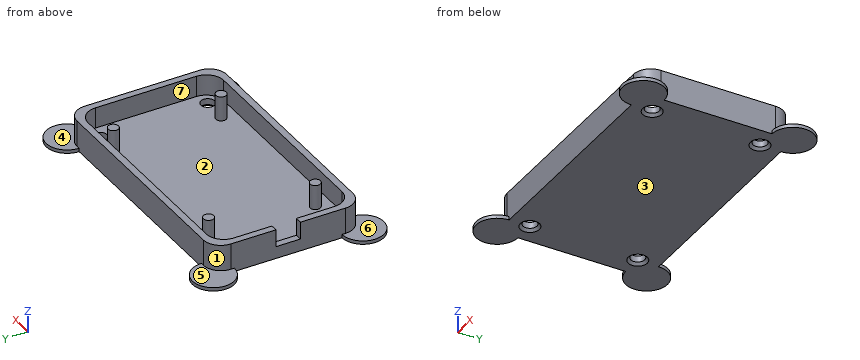
```python
from build123d import *

# Parameters (mm, degrees)
F0_R           = 2
F0_R_2         = 1.5
F0_W           = 2
F0_H           = 7
F1_DEPTH       = 2.5
F2_DEPTH       = 8.5
F3_DEPTH       = 9.6
F4_DEPTH       = 3.5
F5_D           = 3
F5_CSINK_D     = 5.5
F5_CSINK_ANGLE = 90
F6_DEPTH       = 1


with BuildPart() as f1:
    # F0 (on Top) → F1 (new body)
    with BuildSketch(Plane.XY):
        with BuildLine():
            Line((52.2425711751, 68.4110085815), (-6.7574288249, 68.4110085815))
            ThreePointArc((-6.7574288249, 68.4110085815), (-10.2929627308, 66.9465424875), (-11.7574288249, 63.4110085815))
            Line((-11.7574288249, 63.4110085815), (-11.7574288249, 52.4110085815))
            Line((-11.7574288249, 52.4110085815), (-11.7574288249, 45.4110085815))
            Line((-11.7574288249, 45.4110085815), (-11.7574288249, 34.4110085815))
            ThreePointArc((-11.7574288249, 34.4110085815), (-10.2929627308, 30.8754746756), (-6.7574288249, 29.4110085815))
            Line((-6.7574288249, 29.4110085815), (52.2425711751, 29.4110085815))
            ThreePointArc((52.2425711751, 29.4110085815), (55.778105081, 30.8754746756), (57.2425711751, 34.4110085815))
            Line((57.2425711751, 34.4110085815), (57.2425711751, 63.4110085815))
            ThreePointArc((57.2425711751, 63.4110085815), (55.778105081, 66.9465424875), (52.2425711751, 68.4110085815))
        make_face()
        with Locations((-7.7574288249, 33.4110085815)):
            Circle(F0_R, mode=Mode.SUBTRACT)
        with Locations((-1.2574288249, 33.9110085815)):
            Circle(F0_R_2, mode=Mode.SUBTRACT)
        with Locations((45.7425711751, 33.9110085815)):
            Circle(F0_R_2, mode=Mode.SUBTRACT)
        with Locations((53.2425711751, 33.4110085815)):
            Circle(F0_R, mode=Mode.SUBTRACT)
        with Locations((-7.7574288249, 64.4110085815)):
            Circle(F0_R, mode=Mode.SUBTRACT)
        with Locations((-1.8220887287, 64.9110085815)):
            Circle(F0_R_2, mode=Mode.SUBTRACT)
        with Locations((45.7425711751, 64.9110085815)):
            Circle(F0_R_2, mode=Mode.SUBTRACT)
        with Locations((53.2425711751, 64.4110085815)):
            Circle(F0_R, mode=Mode.SUBTRACT)
        with BuildLine():
            ThreePointArc((-11.7574288249, 63.4110085815), (-10.2929627308, 66.9465424875), (-6.7574288249, 68.4110085815))
            Line((-6.7574288249, 68.4110085815), (52.2425711751, 68.4110085815))
            ThreePointArc((52.2425711751, 68.4110085815), (55.778105081, 66.9465424875), (57.2425711751, 63.4110085815))
            Line((57.2425711751, 63.4110085815), (57.2425711751, 34.4110085815))
            ThreePointArc((57.2425711751, 34.4110085815), (55.778105081, 30.8754746756), (52.2425711751, 29.4110085815))
            Line((52.2425711751, 29.4110085815), (-6.7574288249, 29.4110085815))
            ThreePointArc((-6.7574288249, 29.4110085815), (-10.2929627308, 30.8754746756), (-11.7574288249, 34.4110085815))
            Line((-11.7574288249, 34.4110085815), (-11.7574288249, 45.4110085815))
            Line((-11.7574288249, 45.4110085815), (-13.7574288249, 45.4110085815))
            Line((-13.7574288249, 45.4110085815), (-13.7574288249, 33.4110085815))
            Line((-13.7574288249, 33.4110085815), (-13.7574288249, 32.4110085815))
            ThreePointArc((-13.7574288249, 32.4110085815), (-12.2929627308, 28.8754746756), (-8.7574288249, 27.4110085815))
            Line((-8.7574288249, 27.4110085815), (-7.7574288249, 27.4110085815))
            Line((-7.7574288249, 27.4110085815), (53.2425711751, 27.4110085815))
            Line((53.2425711751, 27.4110085815), (54.2425711751, 27.4110085815))
            ThreePointArc((54.2425711751, 27.4110085815), (57.778105081, 28.8754746756), (59.2425711751, 32.4110085815))
            Line((59.2425711751, 32.4110085815), (59.2425711751, 33.4110085815))
            Line((59.2425711751, 33.4110085815), (59.2425711751, 64.4110085815))
            Line((59.2425711751, 64.4110085815), (59.2425711751, 65.4110085815))
            ThreePointArc((59.2425711751, 65.4110085815), (57.778105081, 68.9465424875), (54.2425711751, 70.4110085815))
            Line((54.2425711751, 70.4110085815), (53.2425711751, 70.4110085815))
            Line((53.2425711751, 70.4110085815), (-7.7574288249, 70.4110085815))
            Line((-7.7574288249, 70.4110085815), (-8.7574288249, 70.4110085815))
            ThreePointArc((-8.7574288249, 70.4110085815), (-12.2929627308, 68.9465424875), (-13.7574288249, 65.4110085815))
            Line((-13.7574288249, 65.4110085815), (-13.7574288249, 64.4110085815))
            Line((-13.7574288249, 64.4110085815), (-13.7574288249, 52.4110085815))
            Line((-13.7574288249, 52.4110085815), (-11.7574288249, 52.4110085815))
            Line((-11.7574288249, 52.4110085815), (-11.7574288249, 63.4110085815))
        make_face()
        with Locations((-1.2574288249, 33.9110085815)):
            Circle(F0_R_2)
        with Locations((45.7425711751, 33.9110085815)):
            Circle(F0_R_2)
        with Locations((45.7425711751, 64.9110085815)):
            Circle(F0_R_2)
        with Locations((-1.8220887287, 64.9110085815)):
            Circle(F0_R_2)
        with Locations((-12.7574288249, 48.9110085815)):
            Rectangle(F0_W, F0_H)
    extrude(amount=F1_DEPTH)

    # F0 (on Top) → F2 (join)
    with BuildSketch(Plane.XY):
        with BuildLine():
            ThreePointArc((-11.7574288249, 63.4110085815), (-10.2929627308, 66.9465424875), (-6.7574288249, 68.4110085815))
            Line((-6.7574288249, 68.4110085815), (52.2425711751, 68.4110085815))
            ThreePointArc((52.2425711751, 68.4110085815), (55.778105081, 66.9465424875), (57.2425711751, 63.4110085815))
            Line((57.2425711751, 63.4110085815), (57.2425711751, 34.4110085815))
            ThreePointArc((57.2425711751, 34.4110085815), (55.778105081, 30.8754746756), (52.2425711751, 29.4110085815))
            Line((52.2425711751, 29.4110085815), (-6.7574288249, 29.4110085815))
            ThreePointArc((-6.7574288249, 29.4110085815), (-10.2929627308, 30.8754746756), (-11.7574288249, 34.4110085815))
            Line((-11.7574288249, 34.4110085815), (-11.7574288249, 45.4110085815))
            Line((-11.7574288249, 45.4110085815), (-13.7574288249, 45.4110085815))
            Line((-13.7574288249, 45.4110085815), (-13.7574288249, 33.4110085815))
            Line((-13.7574288249, 33.4110085815), (-13.7574288249, 32.4110085815))
            ThreePointArc((-13.7574288249, 32.4110085815), (-12.2929627308, 28.8754746756), (-8.7574288249, 27.4110085815))
            Line((-8.7574288249, 27.4110085815), (-7.7574288249, 27.4110085815))
            Line((-7.7574288249, 27.4110085815), (53.2425711751, 27.4110085815))
            Line((53.2425711751, 27.4110085815), (54.2425711751, 27.4110085815))
            ThreePointArc((54.2425711751, 27.4110085815), (57.778105081, 28.8754746756), (59.2425711751, 32.4110085815))
            Line((59.2425711751, 32.4110085815), (59.2425711751, 33.4110085815))
            Line((59.2425711751, 33.4110085815), (59.2425711751, 64.4110085815))
            Line((59.2425711751, 64.4110085815), (59.2425711751, 65.4110085815))
            ThreePointArc((59.2425711751, 65.4110085815), (57.778105081, 68.9465424875), (54.2425711751, 70.4110085815))
            Line((54.2425711751, 70.4110085815), (53.2425711751, 70.4110085815))
            Line((53.2425711751, 70.4110085815), (-7.7574288249, 70.4110085815))
            Line((-7.7574288249, 70.4110085815), (-8.7574288249, 70.4110085815))
            ThreePointArc((-8.7574288249, 70.4110085815), (-12.2929627308, 68.9465424875), (-13.7574288249, 65.4110085815))
            Line((-13.7574288249, 65.4110085815), (-13.7574288249, 64.4110085815))
            Line((-13.7574288249, 64.4110085815), (-13.7574288249, 52.4110085815))
            Line((-13.7574288249, 52.4110085815), (-11.7574288249, 52.4110085815))
            Line((-11.7574288249, 52.4110085815), (-11.7574288249, 63.4110085815))
        make_face()
    extrude(amount=F2_DEPTH)

    # F0 (on Top) → F3 (join)
    with BuildSketch(Plane.XY):
        with Locations((-1.8220887287, 64.9110085815)):
            Circle(F0_R_2)
        with Locations((-1.2574288249, 33.9110085815)):
            Circle(F0_R_2)
        with Locations((45.7425711751, 33.9110085815)):
            Circle(F0_R_2)
        with Locations((45.7425711751, 64.9110085815)):
            Circle(F0_R_2)
    extrude(amount=F3_DEPTH)

    # F0 (on Top) → F4 (join)
    with BuildSketch(Plane.XY):
        with Locations((-12.7574288249, 48.9110085815)):
            Rectangle(F0_W, F0_H)
    extrude(amount=F4_DEPTH)

    # F5 (through all)
    with Locations(Plane(origin=(0, 0, 0), x_dir=(1, 0, 0), z_dir=(0, 0, -1))):
        with Locations((53.2425711751, -64.4110085815), (53.2425711751, -33.4110085815), (-7.7574288249, -33.4110085815), (-7.7574288249, -64.4110085815)):
            CounterSinkHole(F5_D / 2, F5_CSINK_D / 2, counter_sink_angle=F5_CSINK_ANGLE)

    # F0 (on Top) → F6 (join)
    with BuildSketch(Plane.XY):
        with BuildLine():
            ThreePointArc((-7.7574288249, 70.4110085815), (-18.000069512, 74.6536492686), (-13.7574288249, 64.4110085815))
            Line((-13.7574288249, 64.4110085815), (-13.7574288249, 65.4110085815))
            ThreePointArc((-13.7574288249, 65.4110085815), (-12.2929627308, 68.9465424875), (-8.7574288249, 70.4110085815))
            Line((-8.7574288249, 70.4110085815), (-7.7574288249, 70.4110085815))
        make_face()
        with BuildLine():
            ThreePointArc((59.2425711751, 64.4110085815), (63.4852118622, 74.6536492686), (53.2425711751, 70.4110085815))
            Line((53.2425711751, 70.4110085815), (54.2425711751, 70.4110085815))
            ThreePointArc((54.2425711751, 70.4110085815), (57.778105081, 68.9465424875), (59.2425711751, 65.4110085815))
            Line((59.2425711751, 65.4110085815), (59.2425711751, 64.4110085815))
        make_face()
        with BuildLine():
            Line((54.2425711751, 27.4110085815), (53.2425711751, 27.4110085815))
            ThreePointArc((53.2425711751, 27.4110085815), (63.4852118622, 23.1683678944), (59.2425711751, 33.4110085815))
            Line((59.2425711751, 33.4110085815), (59.2425711751, 32.4110085815))
            ThreePointArc((59.2425711751, 32.4110085815), (57.778105081, 28.8754746756), (54.2425711751, 27.4110085815))
        make_face()
        with BuildLine():
            Line((-13.7574288249, 32.4110085815), (-13.7574288249, 33.4110085815))
            ThreePointArc((-13.7574288249, 33.4110085815), (-18.000069512, 23.1683678944), (-7.7574288249, 27.4110085815))
            Line((-7.7574288249, 27.4110085815), (-8.7574288249, 27.4110085815))
            ThreePointArc((-8.7574288249, 27.4110085815), (-12.2929627308, 28.8754746756), (-13.7574288249, 32.4110085815))
        make_face()
    extrude(amount=F6_DEPTH)


solid = f1.part
```
CAD build for the part. Positions are in the model's coordinates, mm. Face numbers are marked on the shaded views. A direction names the side the tool comes from. Round coordinates to 2 decimals unless told otherwise and drop trailing zeros. Order: outer loops, then holes, each group sorted by start corner. A loop starts at its lowest first (then second) coordinate and runs counter-clockwise, first axis right, second up.
Q1. Drop flat-ended pins along their axis: pin 1 (13 mm diameter, centred on x = 60, y = 69, fed in from +Z); pin 2 (12 mm diameter, centred on x = 54, y = 68, fed in from -Z); pin 3 (3.5 mm diameter, centred on x = -14.5, y = 72.5, fed in from +Z); pin 4 (1.5 mm diameter, centred on y = 41, z = 7.5, fed in from -X). Give the stop position or say it passes through.
Q2. Two-plate mould, pull along Y, no slides. Class the marked faces 1, 2 and 3: pulls with the +Y half, pulls with the -Y half, needs draft (parallel to the pull), parting line crosses it, or undercut.
Q3. Which spindle directions (+Z, -Z, +X, -X, +Y, -Y) get a long thin tool onto all of the face, cutting with end or side? Do the marked faces 4, 5, 6 and 7. Say none if no direction does.
Q4. Slice it at C-C (z = 7). Write the cut outline in (x, y).
Q5. Wall check: L1, parallel to Y at x = -8, z = 1.25; L2, parallel to Y at x = 17, z = 4.75; L3, parallel to X at y = 39.5, z = 8.25. Give the ranges that are in metal, low to high.
Q6. Slice it at B-B (x = 11). Write the cut outline in (y, z).
Q7. Slice it at A-A (y = 48). Write the cut outline in (x, z).
Results below:
1. pin 1: stops at z = 8.5
1. pin 2: stops at z = 0
1. pin 3: stops at z = 1
1. pin 4: stops at x = -13.76
2. face 1: pulls with the +Y half
2. face 2: undercut
2. face 3: needs draft
3. face 4: +Z, +X, +Y
3. face 5: +Z, -X, +Y
3. face 6: +Z, -X, -Y
3. face 7: +Z
4. outline: (-13.76, 32.41) arc R5 ccw to (-8.76, 27.41) - (54.24, 27.41) arc R5 ccw to (59.24, 32.41) - (59.24, 65.41) arc R5 ccw to (54.24, 70.41) - (-8.76, 70.41) arc R5 ccw to (-13.76, 65.41) - (-13.76, 52.41) - (-11.76, 52.41) - (-11.76, 63.41) arc R5 cw to (-6.76, 68.41) - (52.24, 68.41) arc R5 cw to (57.24, 63.41) - (57.24, 34.41) arc R5 cw to (52.24, 29.41) - (-6.76, 29.41) arc R5 cw to (-11.76, 34.41) - (-11.76, 45.41) - (-13.76, 45.41) - close; circle Ø3 at (-1.82, 64.91); circle Ø3 at (-1.26, 33.91); circle Ø3 at (45.74, 33.91); circle Ø3 at (45.74, 64.91)
5. L1: y = 27.41 to 31.43, 35.4 to 62.43, 66.4 to 70.41
5. L2: y = 27.41 to 29.41, 68.41 to 70.41
5. L3: x = -13.76 to -11.76, 57.24 to 59.24
6. outline: (27.41, 0) - (70.41, 0) - (70.41, 8.5) - (68.41, 8.5) - (68.41, 2.5) - (29.41, 2.5) - (29.41, 8.5) - (27.41, 8.5) - close
7. outline: (-13.76, 0) - (59.24, 0) - (59.24, 8.5) - (57.24, 8.5) - (57.24, 2.5) - (-11.76, 2.5) - (-11.76, 3.5) - (-13.76, 3.5) - close
